```python
from build123d import *

# Parameters (mm, degrees)
SKETCH1_R           = 10
BOSS_EXTRUDE1_DEPTH = 12.5
SKETCH2_R           = 5
CUT_EXTRUDE2_DEPTH  = 8


with BuildPart() as part:
    # Sketch1 → Boss-Extrude1 (new body, symmetric)
    with BuildSketch(Plane.XY):
        Circle(SKETCH1_R)
    extrude(amount=BOSS_EXTRUDE1_DEPTH, both=True)

    # Sketch2 → Cut-Extrude2 (cut)
    with BuildSketch(Plane.XY.offset(12.5)):
        Circle(SKETCH2_R)
    cut_extrude2 = extrude(amount=-CUT_EXTRUDE2_DEPTH, mode=Mode.SUBTRACT)

    # Mirror1: Cut-Extrude2 across plane
    add(cut_extrude2.mirror(Plane.XY), mode=Mode.SUBTRACT)


solid = part.part
```
Check sheet for the modelled part. Datum: model origin and axes. Units: mm. A direction names the side the tool comes from. Round coordinates to 2 decimals unless told otherwise and drop trailing zeros. Loops run counter-clockwise (first coordinate to the right, second up) from the corner with the lowest first, then second, coordinate; pieces in that order, holes last. Notation, with made-up numbers: (-28.5, 68.25) -> (11.5, 68.25) arc R38 cw to (11.5, 106.25) -> close; hole circle Ø7 at (13, -14.75). An arc over 180 degrees is marked (long way). Write item = value, one per line. Start each with the question number.
1) Thickness scan on probe 1 along Y at (x, z) = (0, -7); probe 2 along Z at (x, y) = (1, -0.75); probe 3 along Y at (x, z) = (0.25, 2.25). Record the ranges inside material, lowest first.
2) Sectioned sample at A-A, the plane x = 0. Record the cut outline in (y, z), plus the area to 3 significant figures.
3) Release check for a two-part mould opening along X. For faces 4 (the cylindrical face through (-2.17, -9.76, 0.18)), 5 (the cylindrical face through (-1.08, -4.88, -8.56)), 6 (the cylindrical face through (-1.08, -4.88, 8.56)), 7 (the flat face through (-5, -2, -12.5)) record: released by +X, released by -X, zero draft, split by the parting line, or undercut.
4) Sectioned sample at D-D, the plane z = 3.25. Record the cut outline in (x, y), plus the area to 3 significant figures.
5) Gauge pin test, flat ends, axial feed: pin 1 Ø9 at (x, y) = (0, 0) entering from +Z; pin 2 Ø3 at (x, y) = (-2, 4) entering from -Z; pin 3 Ø8 at (x, z) = (-6, 6.5) entering from -Y; pin 4 Ø3 at (y, z) = (-2, 3.5) entering from -X. Record the tip position at first contact, or that the pin passes through.
6) Set-up check for faces 1 (the flat face through (-5, -2, 12.5)), 2 (the flat face through (0, 0, -4.5)), 3 (the flat face through (0, 0, 4.5)): record each of +Z, -Z, +X, -X, +Y, -Y from which the full face is reachable in a straight line by a thin tool's end or side.
7) Sectioned sample at C-C, the plane z = 10.25. Record the cut outline in (x, y).
Results are:
q1.probe_1 = -10 to -5, 5 to 10
q1.probe_2 = -4.5 to 4.5
q1.probe_3 = -10 to 10
q2.outline = (-10, -12.5) -> (-5, -12.5) -> (-5, -4.5) -> (5, -4.5) -> (5, -12.5) -> (10, -12.5) -> (10, 12.5) -> (5, 12.5) -> (5, 4.5) -> (-5, 4.5) -> (-5, 12.5) -> (-10, 12.5) -> close
q2.area = 340 mm^2
q3.face_4 = split by the parting line
q3.face_5 = undercut
q3.face_6 = undercut
q3.face_7 = zero draft
q4.outline = circle Ø20 at (0, 0)
q4.area = 314 mm^2
q5.pin_1 = 4.5
q5.pin_2 = -12.5
q5.pin_3 = -9.8
q5.pin_4 = -9.99
q6.face_1 = +Z, +X, -X, +Y, -Y
q6.face_2 = -Z
q6.face_3 = +Z
q7.outline = circle Ø20 at (0, 0); hole circle Ø10 at (0, 0)
